Autodesk Inventor part; units mm, degrees
ref_plane "YZ Plane" through (0, 0, 0) normal (1, 0, 0) x (0, 1, 0)
ref_plane "XZ Plane" through (0, 0, 0) normal (0, 1, 0) x (-1, 0, 0)
ref_plane "XY Plane" through (0, 0, 0) normal (0, 0, 1) x (1, 0, 0)
sketch "Sketch1" plane through (0, 0, 0) normal (0, 0, 1) x (1, 0, 0)
  line L0 (-33.02, 52.07) -> (33.02, 52.07)
  line L1 (33.02, 52.07) -> (33.02, -52.07)
  line L2 (33.02, -52.07) -> (-33.02, -52.07)
  line L3 (-33.02, -52.07) -> (-33.02, 52.07)
  line L4 (-42.545, 61.595) -> (42.545, 61.595)
  line L5 (42.545, 61.595) -> (42.545, -61.595)
  line L6 (42.545, -61.595) -> (-42.545, -61.595)
  line L7 (-42.545, -61.595) -> (-42.545, 61.595)
  line L8 (-33.02, 52.07) -> (33.02, 52.07)
  line L9 (33.02, 52.07) -> (33.02, 61.595)
  line L10 (33.02, 61.595) -> (-33.02, 61.595)
  line L11 (-33.02, 61.595) -> (-33.02, 52.07)
  line L12 (-33.02, 52.07) -> (-42.545, 52.07)
  line L13 (-42.545, 52.07) -> (-42.545, -52.07)
  line L14 (-42.545, -52.07) -> (-33.02, -52.07)
  line L15 (-33.02, -52.07) -> (-33.02, 52.07)
  line L16 (33.02, -52.07) -> (42.545, -52.07)
  line L17 (42.545, -52.07) -> (42.545, 52.07)
  line L18 (42.545, 52.07) -> (33.02, 52.07)
  line L19 (33.02, 52.07) -> (33.02, -52.07)
  line L20 (-33.02, -52.07) -> (33.02, -52.07)
  line L21 (33.02, -52.07) -> (33.02, -61.595)
  line L22 (33.02, -61.595) -> (-33.02, -61.595)
  line L23 (-33.02, -61.595) -> (-33.02, -52.07)
  point P0 (0, 0)
  dimension "d0" = 104.14
  dimension "d1" = 123.19
  dimension "d2" = 66.04
  dimension "d3" = 85.09
  dimension "d4" = 52.07
  dimension "d5" = 33.02
  dimension "d6" = 61.595
  dimension "d7" = 42.545
extrude "Extrusion1" add sketch "Sketch1" along normal blind 1.5748 contours L11 L4 L9 L0 | L0 L1 L2 L3 | L3 L14 L7 L12 | L18 L5 L16 L1 | L2 L21 L6 L23
hole "Hole1" at (30.6324, 49.6824, 1.5748) direction (0, 0, -1) diameter 3.175 end through all
hole "Hole2" at (-30.6578, 49.7078, 1.5748) direction (0, 0, -1) diameter 3.175 end through all
hole "Hole3" at (-30.6578, -49.7078, 1.5748) direction (0, 0, -1) diameter 3.175 end through all
hole "Hole4" at (30.6578, -49.7078, 1.5748) direction (0, 0, -1) diameter 3.175 end through all
hole "Hole5" at (10.8712, -43.4848, 1.5748) direction (0, 0, -1) diameter 2.0066 end through all
hole "Hole6" at (-12.4968, 51.8414, 1.5748) direction (0, 0, -1) diameter 3.175 end through all
properties part number "power supply pcb"
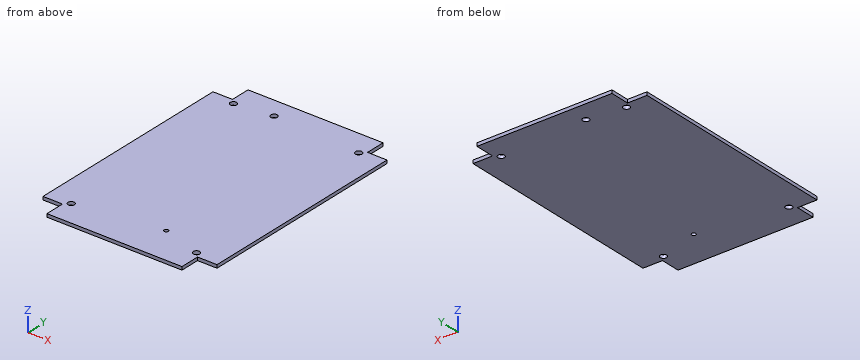
The listing builds one solid part. Answer for the finished solid, in the listing's coordinates (mm). Round coordinates to 2 decimals unless told otherwise and drop trailing zeros. Order: outer loops, then holes, each group sorted by start corner. A loop starts at its lowest first (then second) coordinate and runs counter-clockwise, first axis right, second up. Notation, with made-up numbers: (43, 9.25) -> (101, 9.25) arc R32 cw to (101, 40.25) -> close; hole circle Ø11 at (29, 24.5). An arc over 180 degrees is marked (long way). Put each result on its own line as item: value.
Q1. Consider line 1 along Y through (x, z) = (31, 0.3) (3 decimals); line 2 along X through (y, z) = (-54, 1.15); line 3 along Y through (x, z) = (-12, 0.65) (3 decimals). Determine where each line is inside the solid, lowest interval first.
Results list:
line 1: -61.595 to -51.258, -48.158 to 48.138, 51.227 to 61.595
line 2: -33.02 to 33.02
line 3: -61.595 to 50.334, 53.349 to 61.595
Q2. Section A-A, the plane z = 0.6 is taken. Write down the section's boundary in (x, y) (1 decimal).
Results list:
outline: (-42.5, -52.1) -> (-33, -52.1) -> (-33, -61.6) -> (33, -61.6) -> (33, -52.1) -> (42.5, -52.1) -> (42.5, 52.1) -> (33, 52.1) -> (33, 61.6) -> (-33, 61.6) -> (-33, 52.1) -> (-42.5, 52.1) -> close; hole circle Ø3.2 at (-30.7, -49.7); hole circle Ø3.2 at (-30.7, 49.7); hole circle Ø3.2 at (-12.5, 51.8); hole circle Ø2 at (10.9, -43.5); hole circle Ø3.2 at (30.6, 49.7); hole circle Ø3.2 at (30.7, -49.7)
Q3. Each of these flat-tipped pins is pushed along its axis until it touches: P1, Ø0.5, axis at x = -39, z = 1, coming from the +Y side; P2, Ø1.8, axis at x = 10.87, y = -43.48, coming from the -Z side; P3, Ø0.8, axis at x = 37.5, z = 1, coming from the -Y side. Where does it stop, or does it pass through?
Results list:
P1: y = 52.07
P2: through
P3: y = -52.07
Q4. Section B-B, the plane x = 36.5 is taken. Write down the section's boundary in (y, z).
Results list:
outline: (-52.07, 0) -> (52.07, 0) -> (52.07, 1.57) -> (-52.07, 1.57) -> close
